Input: part model. Units: mm. Frame: model coordinates. A direction names the side the tool comes from. Coordinates: 2 decimals unless noted, no trailing zeros. Loops run counter-clockwise (first coordinate to the right, second up) from the corner with the lowest first, then second, coordinate; pieces in that order, holes last. Notation, with made-up numbers: (25, 38.5) - (53, 38.5) arc R13 cw to (53, 50.5) - close; hole circle Ø1 at (-35.5, 2.5). An arc over 180 degrees is marked (long way). Use one line per item in the form item = value.
from build123d import *

# Parameters (mm, degrees)
F1_DEPTH = 135


with BuildPart() as f1:
    # F0 (on Top) → F1 (new body)
    with BuildSketch(Plane.XY):
        with BuildLine():
            Line((30.371132, 74.60952), (-28.860857, 54.664055))
            Line((-28.860857, 54.664055), (-28.860857, 59.192702))
            ThreePointArc((-28.860857, 59.192702), (-29.543952, 60.909926), (-31.219943, 61.688728))
            ThreePointArc((-31.219943, 61.688728), (-32.895934, 60.909926), (-33.57903, 59.192702))
            Line((-33.57903, 59.192702), (-33.57903, 46.806118))
            ThreePointArc((-33.57903, 46.806118), (-32.846797, 45.038351), (-31.07903, 44.306118))
            Line((-31.07903, 44.306118), (31.16895, 44.306118))
            ThreePointArc((31.16895, 44.306118), (32.936717, 45.038351), (33.66895, 46.806118))
            Line((33.66895, 46.806118), (33.66895, 72.240241))
            ThreePointArc((33.66895, 72.240241), (32.627623, 74.270579), (30.371132, 74.60952))
        make_face()
    extrude(amount=F1_DEPTH)


solid = f1.part
Q1. Pull-direction query (X, two-part tool) for faces 1 (the cylindrical face through (-29.526, 60.891, 66.555)), 2 (the cylindrical face through (32.9, 45, 66.6)), 3 (the flat face through (7, 56, 135)); classes: pulls with the +X half, pulls with the -X half, needs draft (parallel to the pull), parting line crosses it, or undercut.
Check values:
face_1 = undercut
face_2 = pulls with the +X half
face_3 = needs draft
Q2. Ray query, line 1 along X through (y, z) = (46.5, 128.5); line 2 along Y through (x, z) = (-31, 24.5); line 3 along Y through (x, z) = (-4, 81). Return the intervals inside material, ascending. Write a range as [from, to].
Check values:
line_1 = [-33.56, 33.65]
line_2 = [44.31, 61.67]
line_3 = [44.31, 63.04]
Q3. Cut plane D-D, the plane y = 65.5. Return loops of the section in (x, z).
Check values:
outline = (3.32, 0) - (33.67, 0) - (33.67, 135) - (3.32, 135) - close
Q4. Cut plane C-C, the plane x = -21. Return loops of the section in (y, z), then the cut area to 3 significant figures.
Check values:
outline = (44.31, 0) - (57.31, 0) - (57.31, 135) - (44.31, 135) - close
area = 1,760 mm²
Q5. First-contact query: P1, Ø12, axis at x = 5, z = 94, coming from the +Y side; P2, Ø12, axis at x = 2.5, z = 53.5, coming from the +Y side; P3, Ø1.5, axis at x = -15.5, z = 25, coming from the +Y side. Flat tips, straight axial feed; report the tip coordinate or a pass-through.
Check values:
P1 = 68.09
P2 = 67.24
P3 = 59.42
Q6. Cut plane B-B, the plane z = 82.5. Return loops of the section in (x, y), then the cut area to 3 significant figures.
Check values:
outline = (-33.58, 46.81) arc R2.5 ccw to (-31.08, 44.31) - (31.17, 44.31) arc R2.5 ccw to (33.67, 46.81) - (33.67, 72.24) arc R2.5 ccw to (30.37, 74.61) - (-28.86, 54.66) - (-28.86, 59.19) arc R2.5 ccw to (-31.22, 61.69) arc R2.5 ccw to (-33.58, 59.19) - close
area = 1,380 mm²
Q7. Cut plane A-A, the plane y = 56. Return loops of the section in (x, z).
Check values:
outline = (-33.58, 0) - (-28.86, 0) - (-28.86, 135) - (-33.58, 135) - close; (-24.89, 0) - (33.67, 0) - (33.67, 135) - (-24.89, 135) - close
Q8. Set-up query: faces 4 (the flat face through (-28.861, 57, 67)), 5 (the flat face through (-33.579, 53, 67)). Return all of +Z, -Z, +X, -X, +Y, -Y with unobstructed straight access to the full face (end or side cutting, diameter ignored); none if empty.
Check values:
face_4 = +Z, -Z, +Y
face_5 = +Z, -Z, -X, +Y, -Y
